Geometry check sheet. Reference: the model listing, model coordinates, mm. A direction names the side the tool comes from. Coordinates: 2 decimals unless noted, no trailing zeros. Order: outer loops, then holes, each group sorted by start corner. A loop starts at its lowest first (then second) coordinate and runs counter-clockwise, first axis right, second up. Notation, with made-up numbers: (86.5, 1.25) - (99.5, 1.25) arc R11 ccw to (99.5, 13.25) - close; hole circle Ø7 at (-30, 71). An arc over 180 degrees is marked (long way). Return JSON: item names as keys, results as strings. Group by question number.
Item 1: Section check D-D on y = 25. Enter the section's corners in (x, z).
Item 2: Section check A-A on z = 10.5. Enter the section's corners in (x, y), then the cut area to 3 significant figures.
Item 3: Draft check along Y on faces 3 (the cylindrical face through (-0.16, 17.5, 6.26)), 4 (the flat face through (0, -35, 6)), 5 (the flat face through (15, 0, 6)), 6 (the flat face through (0, 35, 6)). Enter one of: pulls with the +Y half, pulls with the -Y half, needs draft (parallel to the pull), parting line crosses it, or undercut.
Item 4: Tool access check on faces 1 (the flat face through (7.5, -5, 6)), 2 (the flat face through (-15, 0, 6)). Record the directions out of +Z, -Z, +X, -X, +Y, -Y that give a thin tool (end or side, any length) a straight path to the whole face; none if there is none.
Item 5: Scan lines: probe 1 along X at (y, z) = (4, 11); probe 2 along X at (y, z) = (27.5, 12); probe 3 along Y at (x, z) = (-2, 6.5). Record each from-to range of solid material in increasing order.
Item 6: Section check C-C on x = 0. Enter the section's corners in (y, z), then the cut area to 4 significant figures.
Item 7: Section check B-B on y = -11. Enter the section's corners in (x, z), then the cut area to 4 significant figures.
from build123d import *

# Parameters (mm, degrees)
CROQUIS1_W              = 30
CROQUIS1_H              = 70
CROQUIS1_R              = 3
SALIENTE_EXTRUIR1_DEPTH = 12.7


with BuildPart() as part:
    # Croquis1 → Saliente-Extruir1 (new body)
    with BuildSketch(Plane.XY):
        Rectangle(CROQUIS1_W, CROQUIS1_H)
        with Locations((-7.5, 25)):
            Circle(CROQUIS1_R, mode=Mode.SUBTRACT)
        with Locations((7.5, 25)):
            Circle(CROQUIS1_R, mode=Mode.SUBTRACT)
        with BuildLine():
            Line((7.5, 10), (7.5, -20))
            ThreePointArc((7.5, -20), (0, -27.5), (-7.5, -20))
            Line((-7.5, -20), (-7.5, 10))
            ThreePointArc((-7.5, 10), (0, 17.5), (7.5, 10))
        make_face(mode=Mode.SUBTRACT)
    extrude(amount=SALIENTE_EXTRUIR1_DEPTH)


solid = part.part
Computed:
{
 "1": {"outline": "(-15, 0) - (-10.5, 0) - (-10.5, 12.7) - (-15, 12.7) - close; (-4.5, 0) - (4.5, 0) - (4.5, 12.7) - (-4.5, 12.7) - close; (10.5, 0) - (15, 0) - (15, 12.7) - (10.5, 12.7) - close"},
 "2": {"outline": "(-15, -35) - (15, -35) - (15, 35) - (-15, 35) - close; hole circle Ø6 at (-7.5, 25); hole (-7.5, -20) arc R7.5 ccw to (7.5, -20) - (7.5, 10) arc R7.5 ccw to (-7.5, 10) - close; hole circle Ø6 at (7.5, 25)", "area": "1,420 mm²"},
 "3": {"face 3": "undercut", "face 4": "pulls with the -Y half", "face 5": "needs draft", "face 6": "pulls with the +Y half"},
 "4": {"face 1": "+Z, -Z", "face 2": "+Z, -Z, -X, +Y, -Y"},
 "5": {"probe 1": "x = -15 to -7.5, 7.5 to 15", "probe 2": "x = -15 to -9.16, -5.84 to 5.84, 9.16 to 15", "probe 3": "y = -35 to -27.23, 17.23 to 35"},
 "6": {"outline": "(-35, 0) - (-27.5, 0) - (-27.5, 12.7) - (-35, 12.7) - close; (17.5, 0) - (35, 0) - (35, 12.7) - (17.5, 12.7) - close", "area": "317.5 mm²"},
 "7": {"outline": "(-15, 0) - (-7.5, 0) - (-7.5, 12.7) - (-15, 12.7) - close; (7.5, 0) - (15, 0) - (15, 12.7) - (7.5, 12.7) - close", "area": "190.5 mm²"}
}
